from build123d import *

# Parameters (mm, degrees)
EXTRUDE_1_DEPTH             = 1.5
SKETCH_2_W                  = 30
SKETCH_2_H                  = 7
EXTRUDE_2_DEPTH             = 117
CUT_EXTRUDE_1_DEPTH         = 93.104529713
CUT_EXTRUDE_2_DEPTH         = 89.933295899
CUT_EXTRUDE_3_DEPTH         = 89.933295899
CUT_EXTRUDE_4_DEPTH         = 93.104529713
HOLE_WIZARD_3_4_3_4_1_D     = 3.4
HOLE_WIZARD_3_4_3_4_1_DEPTH = 7
HOLE_WIZARD_3_4_3_4_2_D     = 3.4
HOLE_WIZARD_3_4_3_4_3_D     = 3.4
HOLE_WIZARD_15_0_15_1_D     = 15
FILLET_1_R                  = 1.5
FILLET_2_R                  = 3
FILLET_3_R                  = 7.5


with BuildPart() as part:
    # 草图1 → 凸台-拉伸1 (new body)
    with BuildSketch(Plane(origin=(0, -32, 0), x_dir=(1, 0, 0), z_dir=(0, 1, 0))):
        with BuildLine():
            Line((-15, 4), (-15, -15.677345132))
            ThreePointArc((-15, -15.677345132), (-13.223342916, -18.57419871), (-9.835839599, -18.303842792))
            ThreePointArc((-9.835839599, -18.303842792), (0, -15.1), (9.835839599, -18.303842792))
            ThreePointArc((9.835839599, -18.303842792), (13.223342916, -18.57419871), (15, -15.677345132))
            Line((15, -15.677345132), (15, 4))
            Line((15, 4), (-15, 4))
        make_face()
    extrude(amount=-EXTRUDE_1_DEPTH)

    # 草图2 → 凸台-拉伸2 (add)
    with BuildSketch(Plane(origin=(0, -32, 0), x_dir=(-1, 0, 0), z_dir=(0, 1, 0))):
        with Locations((0, -0.5)):
            Rectangle(SKETCH_2_W, SKETCH_2_H)
    extrude(amount=EXTRUDE_2_DEPTH)

    # 草图3 → 切除-拉伸1 (cut, through all)
    with BuildSketch(Plane.ZY.offset(15)):
        Polygon((3, 85), (-2.5, 85), (-2.5, 33), (3, 27.5), align=None)
    extrude(amount=-CUT_EXTRUDE_1_DEPTH, mode=Mode.SUBTRACT)

    # 草图4 → 切除-拉伸2 (cut, through all)
    with BuildSketch(Plane.XY.offset(-2.5)):
        with BuildLine():
            Line((-11.795428312, 85), (-15, 85))
            Line((-15, 85), (-15, 60))
            ThreePointArc((-15, 60), (-14.362740383, 64.550068681), (-12.5, 68.75))
            ThreePointArc((-12.5, 68.75), (-10.015546325, 76.782552918), (-11.795428312, 85))
        make_face()
    extrude(amount=-CUT_EXTRUDE_2_DEPTH, mode=Mode.SUBTRACT)

    # 草图5 → 切除-拉伸3 (cut, through all)
    with BuildSketch(Plane.XY.offset(-2.5)):
        with BuildLine():
            Line((15, 85), (11.795428312, 85))
            ThreePointArc((11.795428312, 85), (10.015546325, 76.782552918), (12.5, 68.75))
            ThreePointArc((12.5, 68.75), (14.362740383, 64.550068681), (15, 60))
            Line((15, 60), (15, 85))
        make_face()
    extrude(amount=-CUT_EXTRUDE_3_DEPTH, mode=Mode.SUBTRACT)

    # 草图6 → 切除-拉伸4 (cut, through all)
    with BuildSketch(Plane.ZY.offset(15)):
        Polygon((1.5, -33.5), (1.5, 26.878679656), (-4, 32.378679656), (-4, -33.5), align=None)
    extrude(amount=-CUT_EXTRUDE_4_DEPTH, mode=Mode.SUBTRACT)

    # Ø3.4 (3.4) 直径孔1
    with Locations(Plane.XY.offset(3)):
        with Locations((-5.5, 17.757359313), (5.5, 17.757359313)):
            Hole(HOLE_WIZARD_3_4_3_4_1_D / 2, depth=HOLE_WIZARD_3_4_3_4_1_DEPTH)

    # Ø3.4 (3.4) 直径孔2 (through all)
    with Locations(Plane.XY.offset(-2.5)):
        with Locations((-5.5, 42.5), (5.5, 42.5)):
            Hole(HOLE_WIZARD_3_4_3_4_2_D / 2)

    # Ø3.4 (3.4) 直径孔3 (through all)
    with Locations(Plane(origin=(0, -32, 0), x_dir=(1, 0, 0), z_dir=(0, 1, 0))):
        with Locations((-11.75, -15.677345132), (0, -11.85), (11.75, -15.677345132)):
            Hole(HOLE_WIZARD_3_4_3_4_3_D / 2)

    # Ø15.0 (15) 直径孔1 (through all)
    with Locations(Plane.XY.offset(-2.5)):
        with Locations((0, 75)):
            Hole(HOLE_WIZARD_15_0_15_1_D / 2)

    # 圆角1
    fillet_1_edges = [part.edges().sort_by_distance(p)[0] for p in [
        (0, -32, 3),
        (0, 33, -2.5),
        (0, 26.878679656, 1.5),
    ]]
    fillet(fillet_1_edges, radius=FILLET_1_R)

    # 圆角2
    fillet_2_edges = [part.edges().sort_by_distance(p)[0] for p in [
        (0, 27.5, 3),
        (0, -33.5, 1.5),
        (0, 32.378679656, -4),
    ]]
    fillet(fillet_2_edges, radius=FILLET_2_R)

    # 圆角3
    fillet_3_edges = [part.edges().sort_by_distance(p)[0] for p in [
        (-11.795428312, 85, -3.25),
        (11.795428312, 85, -3.25),
    ]]
    fillet(fillet_3_edges, radius=FILLET_3_R)


solid = part.part
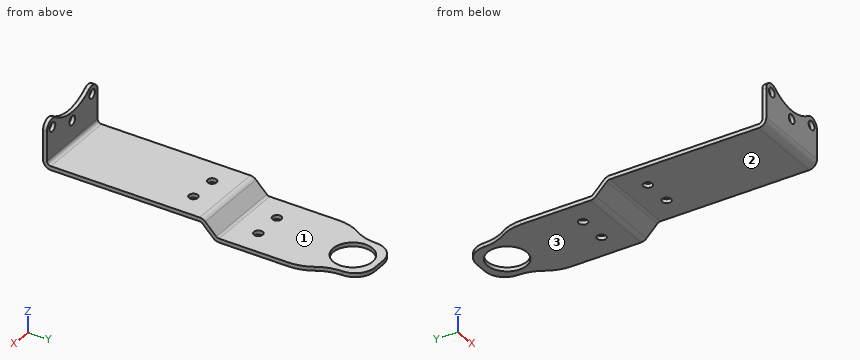
Geometry: final body of the model. Coordinates: model frame, mm. Face numbers are marked on the shaded views. A direction names the side the tool comes from. Coordinates: 2 decimals unless noted, no trailing zeros. Order: outer loops, then holes, each group sorted by start corner. A loop starts at its lowest first (then second) coordinate and runs counter-clockwise, first axis right, second up.
(1) First-contact query: pin 1 (5 mm diameter, centred on x = -2.5, y = 21, fed in from -Z); pin 2 (2 mm diameter, centred on x = -5.5, y = 42.5, fed in from -Z); pin 3 (15 mm diameter, centred on x = -2.5, y = 71.5, fed in from +Z); pin 4 (7 mm diameter, centred on x = 3, z = 11.5, fed in from +Y). Flat tips, straight axial feed; report the tip coordinate or a pass-through.
(2) Section query C-C (x = -6). Return the cut outline in (y, z), plus the area to 3 significant figures.
(3) Material intervals for probe 1 along Z at (x, y) = (7, -5); probe 2 along Z at (x, y) = (0, -32.8); probe 3 along X at (y, z) = (-32.95, 11.85), sorted ascending.
(4) Access query for the marked faces 1, 2 and 3. Directions: +Z, -Z, +X, -X, +Y, -Y. A direction counts if a zero-diameter tool reaches every point of the face in a straight line with its end or side. Return the directions, or none.
(5) Section query D-D (y = 75). Return the cut outline in (x, z), plus the area to 3 significant figures.
(6) Section query B-B (y = 42.5). Return the cut outline in (x, z), plus the area to 3 significant figures.
(7) Section query A-A (z = 11.85). Return the cut outline in (x, y), plus the area to 3 significant figures.
Solution:
1. pin 1: stops at z = 1.5
1. pin 2: passes through
1. pin 3: stops at z = -2.5
1. pin 4: stops at y = -32
2. outline: (-33.5, 4.5) arc R3 ccw to (-30.5, 1.5) - (16.13, 1.5) - (16.13, 3) - (-30.5, 3) arc R1.5 cw to (-32, 4.5) - (-32, 16.22) - (-33.5, 16.22) - close; (19.38, 1.5) - (26.26, 1.5) arc R1.5 cw to (27.32, 1.06) - (31.5, -3.12) arc R3 ccw to (33.62, -4) - (40.88, -4) - (40.88, -2.5) - (33.62, -2.5) arc R1.5 cw to (32.56, -2.06) - (28.38, 2.12) arc R3 ccw to (26.26, 3) - (19.38, 3) - close; (44.12, -4) - (70.5, -4) - (70.5, -2.5) - (44.12, -2.5) - close; (79.5, -4) - (84.13, -4) - (84.13, -2.5) - (79.5, -2.5) - close
2. area: 175 mm2
3. probe 1: z = 1.5 to 3
3. probe 2: z = 2.57 to 10.15, 13.55 to 15.1
3. probe 3: x = -15 to -1.7, 1.7 to 15
4. face 1: +Z, +X, -X, +Y
4. face 2: -Z, +X, -X, -Y
4. face 3: -Z, +X, -X, +Y, -Y
5. outline: (-10.19, -4) - (-7.5, -4) - (-7.5, -2.5) - (-10.19, -2.5) - close; (7.5, -4) - (10.19, -4) - (10.19, -2.5) - (7.5, -2.5) - close
5. area: 8.07 mm2
6. outline: (-15, -4) - (-7.2, -4) - (-7.2, -2.5) - (-15, -2.5) - close; (-3.8, -4) - (3.8, -4) - (3.8, -2.5) - (-3.8, -2.5) - close; (7.2, -4) - (15, -4) - (15, -2.5) - (7.2, -2.5) - close
6. area: 34.8 mm2
7. outline: (-15, -33.5) - (-1.7, -33.5) - (-1.7, -32) - (-15, -32) - close; (1.7, -33.5) - (15, -33.5) - (15, -32) - (1.7, -32) - close
7. area: 39.9 mm2
